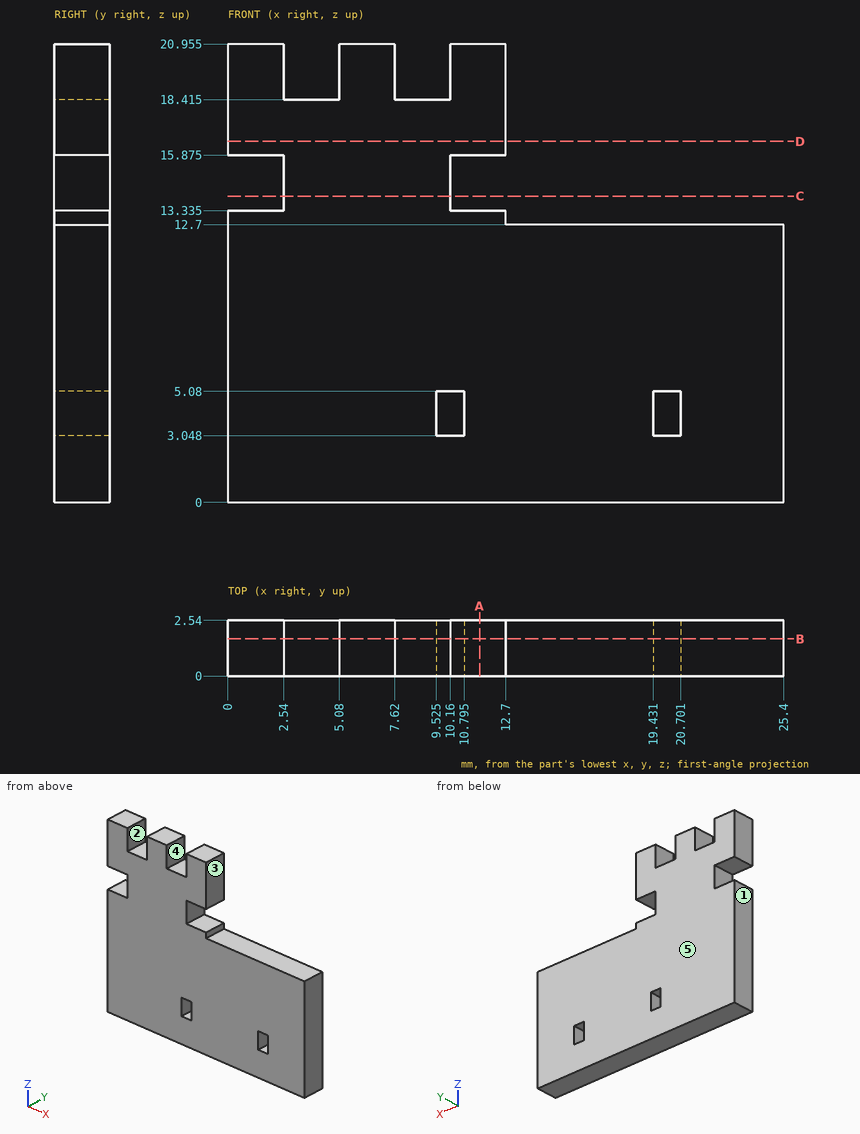
Source: three-view drawing plus pictorial views. Frame: mm from the lowest corner of the part. A direction names the side the tool comes from. Coordinates: 2 decimals unless noted, no trailing zeros. Write each loop counter-clockwise with the first axis right and the second up, starting at its lowest first coordinate (ties: lowest second). Pieces come first, ordered by that corner, then holes. Notation, with made-up numbers: (11, 68) - (51, 68) arc R20 cw to (51, 96) - close; hole circle Ø5 at (-33, 34). An arc over 180 degrees is marked (long way). Return JSON: item names as keys, results as strings.
Item 1: Section query B-B (y = 1.7). Count the separate pieces of the cut face and the enclosed holes in it, and give its area (3 significant figures).
Completed:
{"separate pieces": "1", "enclosed holes": "2", "area": "396 mm2"}
Item 2: Section query A-A (x = 11.5). Output: boundary loops of the cut face in (y, z) (3 decimals), and give its area (3 significant figures).
Completed:
{"outline": "(0, 0) - (2.54, 0) - (2.54, 13.335) - (0, 13.335) - close; (0, 15.875) - (2.54, 15.875) - (2.54, 20.955) - (0, 20.955) - close", "area": "46.8 mm2"}
Item 3: Pull-direction query (X, two-part tool) for the marked faces 1, 2 and 3; classes: +X half, -X half, draft (parallel to the pull), parting line (faces both ways), or undercut.
Completed:
{"face 1": "-X half", "face 2": "undercut", "face 3": "+X half"}
Item 4: Line query: L1, parallel to X at y = 1.5, z = 19.25; L2, parallel to X at y = 0.15, z = 3.75 (3 decimals); L3, parallel to Z at x = 21.25, y = 0.3. Output: solid intervals per line, ascending.
Completed:
{"L1": "x = 0 to 2.54, 5.08 to 7.62, 10.16 to 12.7", "L2": "x = 0 to 9.525, 10.795 to 19.431, 20.701 to 25.4", "L3": "z = 0 to 12.7"}
Item 5: Section query C-C (z = 14). Output: boundary loops of the cut face in (x, y).
Completed:
{"outline": "(2.54, 0) - (10.16, 0) - (10.16, 2.54) - (2.54, 2.54) - close"}
Item 6: Pin query (flat end, axial travel): pin 1 Ø0.8 at (y, z) = (1, 14) entering from -X; pin 2 Ø1.3 at (y, z) = (1.5, 14.5) entering from +X; pin 3 Ø1.3 at (y, z) = (1.5, 18.5) entering from +X. Return the tip coordinate at first contact, or that it passes through.
Completed:
{"pin 1": "stops at x = 2.54", "pin 2": "stops at x = 10.16", "pin 3": "stops at x = 12.7"}
Item 7: Reachability of the marked faces 4 and 5 from +Z, -Z, +X, -X, +Y, -Y: full face, straight path, thin tool, end or side. Return the list, or none.
Completed:
{"face 4": "+Z, +Y, -Y", "face 5": "+Z, -Z, +X, -X, +Y"}
Item 8: Section query D-D (z = 16.5). Output: boundary loops of the cut face in (x, y), and give its area (3 significant figures).
Completed:
{"outline": "(0, 0) - (12.7, 0) - (12.7, 2.54) - (0, 2.54) - close", "area": "32.3 mm2"}
